```python
from build123d import *

# Parameters (mm, degrees)
BOSS_EXTRU_2_DEPTH = 32
CONG_2_R           = 2


with BuildPart() as part:
    # Esquisse1 → Boss.-Extru.2 (new body)
    with BuildSketch(Plane.XY):
        with BuildLine():
            Line((33.25, 68), (33.25, 34))
            Line((33.25, 34), (33.25, 0))
            Line((33.25, 0), (0, 0))
            Line((0, 0), (0, -0.4))
            Line((0, -0.4), (33.65, -0.4))
            Line((33.65, -0.4), (33.65, 34))
            Line((33.65, 34), (33.65, 68))
            ThreePointArc((33.65, 68), (28.572164781, 71.359134798), (27.46710324, 65.37189536))
            Line((27.46710324, 65.37189536), (27.75, 65.65479212))
            ThreePointArc((27.75, 65.65479212), (28.725245122, 70.989565186), (33.25, 68))
        make_face()
    extrude(amount=BOSS_EXTRU_2_DEPTH)

    # Congé2
    cong_2_edges = [part.edges().sort_by_distance(p)[0] for p in [
        (33.25, 0, 16),
        (33.65, -0.4, 16),
    ]]
    fillet(cong_2_edges, radius=CONG_2_R)

    # Symétrie2: part across plane


with BuildPart() as part_1:
    add(part.part)
    add(part.part.mirror(Plane(origin=(0, -0.4, 32), x_dir=(0, 0, 1), z_dir=(1, 0, 0))))


solid = part_1.part
```
Here's how the part is built. I have some questions about the finished solid (model axes, mm). A direction names the side the tool comes from. Give positions to 0.01 mm unless a question says otherwise; leave off trailing zeros. Order: outer loops, then holes, each group sorted by start corner. A loop starts at its lowest first (then second) coordinate and runs counter-clockwise, first axis right, second up. Notation, with made-up numbers: (-19.75, 49) - (12.25, 49) arc R13 ccw to (12.25, 67) - close; hole circle Ø4 at (-5.5, 87.25). An arc over 180 degrees is marked (long way). Answer as a JSON object with one key per item and string values. Group by question number.
Item 1: If we mould it in two halves opening along X, with no side actions, what happens to faces 3 (the cylindrical face through (-28.67, 71.4, 15.78)), 4 (the flat face through (33.65, 34, 16)), 5 (the flat face through (-33.65, 34, 16)), 6 (the flat face through (0, -0.4, 16))? For each: pulls with the +X half, pulls with the -X half, needs draft (parallel to the pull), parting line crosses it, or undercut.
Item 2: If we section it at A-A on y = 31.5: Please give me the cut outline in (x, z).
Item 3: For P1, Ø12, axis at x = -22.5, y = 49.5, coming from the -Z side; P2, Ø10.5, axis at x = 30, y = 68, coming from the +Z side; P3, Ø16, axis at x = -14.5, z = 23.5, coming from the +Y side, each with a flat end and sliding along its axis, tell me the tip position at first contact or that it passes through.
Item 4: Please list where these lines run through material, in increasing order: probe 1 along X at (y, z) = (68, 24); probe 2 along Y at (x, z) = (30, 12); probe 3 along X at (y, z) = (44, 17.5).
Item 5: If we section it at C-C on x = 30: Please give me the cut outline in (y, z), and give its area (3 significant figures).
Item 6: Which directions (+Z, -Z, +X, -X, +Y, -Y) give clear straight access to the entire face, cutting with the end or side of a thin tool? Please do faces 1 (the flat face through (-33.25, 35, 16)), 2 (the cylindrical face through (-33.05, 0.17, 16.22)).
Item 7: If we section it at D-D on x = -8: Please give me the cut outline in (y, z).
Item 8: If we section it at B-B on z = 13: Please give me the cut outline in (x, y).
Result set:
{
 "1": {"face 3": "undercut", "face 4": "pulls with the +X half", "face 5": "pulls with the -X half", "face 6": "needs draft"},
 "2": {"outline": "(-33.65, 0) - (-33.25, 0) - (-33.25, 32) - (-33.65, 32) - close; (33.25, 0) - (33.65, 0) - (33.65, 32) - (33.25, 32) - close"},
 "3": {"P1": "through", "P2": "z = 32", "P3": "y = 0"},
 "4": {"probe 1": "-33.65 to -33.25, -26.75 to -26.35, 26.35 to 26.75, 33.25 to 33.65", "probe 2": "-0.4 to 0, 71.25 to 71.65", "probe 3": "-33.65 to -33.25, 33.25 to 33.65"},
 "5": {"outline": "(-0.4, 0) - (0, 0) - (0, 32) - (-0.4, 32) - close; (71.25, 0) - (71.65, 0) - (71.65, 32) - (71.25, 32) - close", "area": "25.6 mm²"},
 "6": {"face 1": "+Z, -Z", "face 2": "+Z, -Z, -X, -Y"},
 "7": {"outline": "(-0.4, 0) - (0, 0) - (0, 32) - (-0.4, 32) - close"},
 "8": {"outline": "(-33.65, 1.6) arc R2 ccw to (-31.65, -0.4) - (31.65, -0.4) arc R2 ccw to (33.65, 1.6) - (33.65, 68) arc R3.65 ccw (long way) to (27.47, 65.37) - (27.75, 65.65) arc R3.25 cw (long way) to (33.25, 68) - (33.25, 2) arc R2 cw to (31.25, 0) - (-31.25, 0) arc R2 cw to (-33.25, 2) - (-33.25, 68) arc R3.25 cw (long way) to (-27.75, 65.65) - (-27.47, 65.37) arc R3.65 ccw (long way) to (-33.65, 68) - close"}
}
